Design review of the part built by this model. Coordinates are the model's own, in mm. Coordinates: 2 decimals unless noted, no trailing zeros. Write item = value, one per line.
```python
from build123d import *

# Parameters (mm, degrees)
SKETCH1_W                  = 15.875
SKETCH1_H                  = 6.35
BOSS_EXTRUDE1_DEPTH        = 1803.4
TAP_DRILL_FOR_10_32_TAP1_D = 4.0386


with BuildPart() as part:
    # Sketch1 → Boss-Extrude1 (new body)
    with BuildSketch(Plane(origin=(0, 0, 0), x_dir=(1, 0, 0), z_dir=(0, 1, 0))):
        with Locations((7.9375, 3.175)):
            Rectangle(SKETCH1_W, SKETCH1_H)
    extrude(amount=BOSS_EXTRUDE1_DEPTH)

    # Tap Drill for #10-32 Tap1 (through all)
    with Locations(Plane.XY):
        with Locations((7.9375, 12.7), (7.9375, 44.45), (7.9375, 57.15), (7.9375, 88.9), (7.9375, 101.6), (7.9375, 133.35), (7.9375, 146.05), (7.9375, 177.8), (7.9375, 190.5), (7.9375, 222.25), (7.9375, 234.95), (7.9375, 266.7), (7.9375, 279.4), (7.9375, 311.15), (7.9375, 323.85), (7.9375, 355.6), (7.9375, 368.3), (7.9375, 400.05), (7.9375, 412.75), (7.9375, 444.5), (7.9375, 457.2), (7.9375, 488.95), (7.9375, 501.65), (7.9375, 533.4), (7.9375, 546.1), (7.9375, 577.85), (7.9375, 590.55), (7.9375, 622.3), (7.9375, 635), (7.9375, 666.75), (7.9375, 679.45), (7.9375, 711.2), (7.9375, 723.9), (7.9375, 755.65), (7.9375, 768.35), (7.9375, 800.1), (7.9375, 812.8), (7.9375, 844.55), (7.9375, 857.25), (7.9375, 889), (7.9375, 901.7), (7.9375, 933.45), (7.9375, 946.15), (7.9375, 977.9), (7.9375, 990.6), (7.9375, 1022.35), (7.9375, 1035.05), (7.9375, 1066.8), (7.9375, 1079.5), (7.9375, 1111.25), (7.9375, 1123.95), (7.9375, 1155.7), (7.9375, 1168.4), (7.9375, 1200.15), (7.9375, 1212.85), (7.9375, 1244.6), (7.9375, 1257.3), (7.9375, 1289.05), (7.9375, 1301.75), (7.9375, 1333.5), (7.9375, 1346.2), (7.9375, 1377.95), (7.9375, 1390.65), (7.9375, 1422.4), (7.9375, 1435.1), (7.9375, 1466.85), (7.9375, 1479.55), (7.9375, 1511.3), (7.9375, 1524), (7.9375, 1555.75), (7.9375, 1568.45), (7.9375, 1600.2), (7.9375, 1612.9), (7.9375, 1644.65), (7.9375, 1657.35), (7.9375, 1689.1), (7.9375, 1701.8), (7.9375, 1733.55), (7.9375, 1746.25), (7.9375, 1778)):
            Hole(TAP_DRILL_FOR_10_32_TAP1_D / 2)


solid = part.part
```
(1) We need section A-A (z = -2.5). Give the number of separate pieces and of enclosed holes in the cut face, and give its area (3 significant figures).
Report:
separate_pieces = 1
enclosed_holes = 80
area = 27,600 mm²
(2) Insertion check: pin 1 (2 mm diameter, centred on x = 14.5, z = -4, fed in from -Y); pin 2 (2.5 mm diameter, centred on x = 7.94, y = 133.35, fed in from +Z). Each pin has a flat end and moves straight along its axis. Give the tip position at first contact, or say it passes through.
Report:
pin_1 = 0
pin_2 = through
(3) For L1, parallel to X at y = 1701.5, z = -2 (3 decimals); L2, parallel to X at y = 488.95, z = -3 (3 decimals), list the stretches that pass through material, from the lowest coordinate up.
Report:
L1 = 0 to 5.941, 9.934 to 15.875
L2 = 0 to 5.918, 9.957 to 15.875
